Design review of the part built by this model. Coordinates are the model's own, in mm. A direction names the side the tool comes from. Round coordinates to 2 decimals unless told otherwise and drop trailing zeros. Loops run counter-clockwise (first coordinate to the right, second up) from the corner with the lowest first, then second, coordinate; pieces in that order, holes last. Notation, with made-up numbers: M 74.25,-22 L 131.25,-22 A22 cw 131.25,-14 Z; hole C 37.25,39 d7. An arc over 180 degrees is marked long. One line per item, written item: value. Start each with the question number.
Item 1: Mouldability with a two-part tool opening along X and no side actions: class faces 4 (the flat face through (-23, 2, 27)), 5 (the cylindrical face through (-2.85, 51.99, 32.04)), 6 (the flat face through (-28, 53, 32)) as released by +X, released by -X, zero draft, split by the parting line, or undercut.
Item 2: We need section C-C (z = 57.5). Write out the cut boundary in (x, y), then the cut area to 3 significant figures.
Item 3: We need section B-B (x = -81.5). Write out the cut boundary in (y, z), then the cut area to 3 significant figures.
Item 4: We need section D-D (y = 16.5). Write out the cut boundary in (x, z), then the cut area to 3 significant figures.
Item 5: Clearance check with flat-ended pins moving along their axes: pin 1 (9 mm diameter, centred on x = -19, z = 55, fed in from +Y); pin 2 (17.5 mm diameter, centred on y = 30, z = 24.5, fed in from -X); pin 3 (2 mm diameter, centred on y = 54, z = 17, fed in from -X). State where each tip first meets the part, or that it passes through.
Item 6: For faces 1 (the cylindrical face through (-5.711, 5.804, 32.045)), 2 (the flat face through (-22, 2, 38)), 3 (the cylindrical face through (-18.349, 53.028, 59.957)), list the 3-axis set-ups (+Z, -Z, +X, -X, +Y, -Y) from which the entire face can be reached by the end or side of a thin tool; tool diameter is ignored.
Item 7: For line 1 along Z through (x, y) = (-19, 53); line 2 along Y through (x, z) = (-22, 19.5); line 3 along Y through (x, z) = (-32, 14), list the stretches that pass through material, from the lowest coordinate up.
Item 8: We need section A-A (z = 12). Write out the cut boundary in (x, y), then the cut area to 3 significant figures.
from build123d import *

# Parameters (mm, degrees)
F1_DEPTH  = 65
F3_R      = 34
F4_DEPTH  = 25
F5_R      = 1
F7_R      = 5
F8_DEPTH  = 25
F11_DEPTH = 25


with BuildPart() as f1:
    # F0 (on Top) → F1 (new body)
    with BuildSketch(Plane.XY):
        with BuildLine():
            ThreePointArc((-10, 0), (-2.9289321881, 2.9289321881), (0, 10))
            Line((0, 10), (0, 45))
            ThreePointArc((0, 45), (-2.9289321881, 52.0710678119), (-10, 55))
            Line((-10, 55), (-28, 55))
            Line((-28, 55), (-28, 51))
            Line((-28, 51), (-10, 51))
            ThreePointArc((-10, 51), (-5.7573593129, 49.2426406871), (-4, 45))
            Line((-4, 45), (-4, 10))
            ThreePointArc((-4, 10), (-5.7573593129, 5.7573593129), (-10, 4))
            Line((-10, 4), (-110, 4))
            Line((-110, 4), (-110, 0))
            Line((-110, 0), (-10, 0))
        make_face()
    extrude(amount=F1_DEPTH)

    # F3 (on offset) → F4 (cut)
    with BuildSketch(Plane(origin=(0, 4, 0), x_dir=(-1, 0, 0), z_dir=(0, 1, 0))):
        with Locations((110, 32.5)):
            Circle(F3_R)
    extrude(amount=-F4_DEPTH, mode=Mode.SUBTRACT)

    # F5
    f5_edges = [f1.edges().sort_by_distance(p)[0] for p in [
        (-100.012508, 2, 65),
        (-100.012508, 2, 0),
    ]]
    fillet(f5_edges, radius=F5_R)

    # F7 (on offset) → F8 (cut)
    with BuildSketch(Plane(origin=(0, 55, 0), x_dir=(-1, 0, 0), z_dir=(0, 1, 0))):
        with Locations((19, 55)):
            Circle(F7_R)
        with Locations((19, 10)):
            Circle(F7_R)
    extrude(amount=-F8_DEPTH, mode=Mode.SUBTRACT)

    # F10 (on offset) → F11 (cut)
    with BuildSketch(Plane.XZ):
        with BuildLine():
            Line((-27, 27), (-18, 27))
            ThreePointArc((-18, 27), (-14.1109127035, 28.6109127035), (-12.5, 32.5))
            ThreePointArc((-12.5, 32.5), (-14.1109127035, 36.3890872965), (-18, 38))
            Line((-18, 38), (-27, 38))
            ThreePointArc((-27, 38), (-30.8890872965, 36.3890872965), (-32.5, 32.5))
            ThreePointArc((-32.5, 32.5), (-30.8890872965, 28.6109127035), (-27, 27))
        make_face()
    extrude(amount=-F11_DEPTH, mode=Mode.SUBTRACT)


solid = f1.part
A:
1. face 4: undercut
1. face 5: released by +X
1. face 6: released by -X
2. outline: M -86.96,0 L -10,0 A10 ccw 0,10 L 0,45 A10 ccw -10,55 L -14.67,55 L -14.67,51 L -10,51 A6 cw -4,45 L -4,10 A6 cw -10,4 L -86.96,4 Z; M -28,51 L -23.33,51 L -23.33,55 L -28,55 Z
2. area: 586 mm2
3. outline: M 0,0 L 4,0 L 4,13.96 L 0,13.96 Z; M 0,51.04 L 4,51.04 L 4,65 L 0,65 Z
3. area: 112 mm2
4. outline: M -4,0 L 0,0 L 0,65 L -4,65 Z
4. area: 260 mm2
5. pin 1: y = 4
5. pin 2: x = -4
5. pin 3: x = -28
6. face 1: +Z, -Z, -X
6. face 2: -Y
6. face 3: +Y
7. line 1: 0 to 5, 15 to 50, 60 to 65
7. line 2: 0 to 4, 51 to 55
7. line 3: 0 to 4
8. outline: M -82.88,0 L -10,0 A10 ccw 0,10 L 0,45 A10 ccw -10,55 L -14.42,55 L -14.42,51 L -10,51 A6 cw -4,45 L -4,10 A6 cw -10,4 L -82.88,4 Z; M -28,51 L -23.58,51 L -23.58,55 L -28,55 Z
8. area: 567 mm2
